from build123d import *

# Parameters (mm, degrees)
SKETCH_1_R          = 2
SKETCH_1_W          = 3
SKETCH_1_H          = 10
EXTRUDE_1_DEPTH     = 3
SKETCH_2_W          = 3
SKETCH_2_H          = 60
EXTRUDE_2_DEPTH     = 31
SKETCH_3_W          = 25
SKETCH_3_H          = 3
EXTRUDE_3_DEPTH     = 5
SKETCH_4_W          = 10
SKETCH_4_H          = 3
SKETCH_4_W_2        = 6
SKETCH_4_W_3        = 3
SKETCH_4_H_2        = 10
CUT_EXTRUDE_1_DEPTH = 3
SKETCH_5_R          = 1
CUT_EXTRUDE_2_DEPTH = 3
FILLET_1_R          = 1


with BuildPart() as part:
    # 草图1 → 凸台-拉伸1 (new body)
    with BuildSketch(Plane.XY):
        Polygon((-5, 25), (-5, 28), (1, 28), (1, 25), (5, 25), (10, 25), (20, 25), (25, 25), (30, 25), (30, -25), (25, -25), (20, -25), (10, -25), (5, -25), (1, -25), (1, -28), (-5, -28), (-5, -25), (-9, -25), (-9, -28), (-15, -28), (-15, -25), (-20, -25), (-20, 25), (-15, 25), (-15, 28), (-9, 28), (-9, 25), align=None)
        with Locations((-11, 15)):
            Circle(SKETCH_1_R, mode=Mode.SUBTRACT)
        with Locations((-11, -15)):
            Circle(SKETCH_1_R, mode=Mode.SUBTRACT)
        with Locations((19, -15)):
            Circle(SKETCH_1_R, mode=Mode.SUBTRACT)
        with Locations((19, 15)):
            Circle(SKETCH_1_R, mode=Mode.SUBTRACT)
        with Locations((26.5, 15)):
            Rectangle(SKETCH_1_W, SKETCH_1_H, mode=Mode.SUBTRACT)
        with Locations((26.5, 0)):
            Rectangle(SKETCH_1_W, SKETCH_1_H, mode=Mode.SUBTRACT)
        with Locations((26.5, -15)):
            Rectangle(SKETCH_1_W, SKETCH_1_H, mode=Mode.SUBTRACT)
        with Locations((1.5, 0)):
            Rectangle(SKETCH_1_W, SKETCH_1_H, mode=Mode.SUBTRACT)
        with Locations((1.5, -15)):
            Rectangle(SKETCH_1_W, SKETCH_1_H, mode=Mode.SUBTRACT)
        with Locations((1.5, 15)):
            Rectangle(SKETCH_1_W, SKETCH_1_H, mode=Mode.SUBTRACT)
    extrude(amount=EXTRUDE_1_DEPTH)

    # 草图2 → 凸台-拉伸2 (add)
    with BuildSketch(Plane.ZY.offset(20)):
        with Locations((1.5, 0)):
            Rectangle(SKETCH_2_W, SKETCH_2_H)
    extrude(amount=EXTRUDE_2_DEPTH)

    # 草图3 → 凸台-拉伸3 (add)
    with BuildSketch(Plane(origin=(0, 25, 0), x_dir=(1, 0, 0), z_dir=(0, 1, 0))):
        with Locations((17.5, -1.5)):
            Rectangle(SKETCH_3_W, SKETCH_3_H)
    extrude_3 = extrude(amount=EXTRUDE_3_DEPTH)

    # 镜向1: 凸台-拉伸3 across plane
    add(extrude_3.mirror(Plane.ZX))

    # 草图4 → 切除-拉伸1 (cut)
    with BuildSketch(Plane.XY.offset(3)):
        with Locations((-43, 26.5)):
            Rectangle(SKETCH_4_W, SKETCH_4_H)
        with Locations((-29, 26.5)):
            Rectangle(SKETCH_4_W, SKETCH_4_H)
        with Locations((12, 26.5)):
            Rectangle(SKETCH_4_W_2, SKETCH_4_H)
        with Locations((22, 26.5)):
            Rectangle(SKETCH_4_W_2, SKETCH_4_H)
        with Locations((22, -26.5)):
            Rectangle(SKETCH_4_W_2, SKETCH_4_H)
        with Locations((12, -26.5)):
            Rectangle(SKETCH_4_W_2, SKETCH_4_H)
        with Locations((-29, -26.5)):
            Rectangle(SKETCH_4_W, SKETCH_4_H)
        with Locations((-43, -26.5)):
            Rectangle(SKETCH_4_W, SKETCH_4_H)
        with Locations((-47.5, 0)):
            Rectangle(SKETCH_4_W_3, SKETCH_4_H_2)
        with Locations((-47.5, 15)):
            Rectangle(SKETCH_4_W_3, SKETCH_4_H_2)
        with Locations((-47.5, -15)):
            Rectangle(SKETCH_4_W_3, SKETCH_4_H_2)
    extrude(amount=-CUT_EXTRUDE_1_DEPTH, mode=Mode.SUBTRACT)

    # 草图5 → 切除-拉伸2 (cut)
    with BuildSketch(Plane(origin=(0, 0, 0), x_dir=(-1, 0, 0), z_dir=(0, 0, -1))):
        with Locations((23, 22.6)):
            Circle(SKETCH_5_R)
        with Locations((41, 22.6)):
            Circle(SKETCH_5_R)
        with Locations((41, -22.6)):
            Circle(SKETCH_5_R)
        with Locations((23, -22.6)):
            Circle(SKETCH_5_R)
        with BuildLine():
            Line((2, 7.351919832), (2, -7.055869369))
            Line((2, -7.055869369), (2, -10.9658561))
            ThreePointArc((2, -10.9658561), (8.5, 0), (2, 10.9658561))
            Line((2, 10.9658561), (2, 7.351919832))
        make_face()
        Polygon((23, -15), (23, 15), (28.973451327, 0), align=None)
        Polygon((27, -20), (32, -7.444444444), (37, -20), align=None)
        Polygon((41, -15), (35.026548673, 0), (41, 15), align=None)
        Polygon((27, 20), (37, 20), (32, 7.444444444), align=None)
    extrude(amount=-CUT_EXTRUDE_2_DEPTH, mode=Mode.SUBTRACT)

    # 圆角1
    fillet_1_edges = [part.edges().sort_by_distance(p)[0] for p in [
        (-2, 10.9658561, 1.5),
        (-2, -10.9658561, 1.5),
        (-23, 15, 1.5),
        (-28.973451327, 0, 1.5),
        (-23, -15, 1.5),
        (-37, 20, 1.5),
        (-32, 7.444444444, 1.5),
        (-27, 20, 1.5),
        (-41, 15, 1.5),
        (-41, -15, 1.5),
        (-35.026548673, 0, 1.5),
        (-37, -20, 1.5),
        (-27, -20, 1.5),
        (-32, -7.444444444, 1.5),
    ]]
    fillet(fillet_1_edges, radius=FILLET_1_R)


solid = part.part
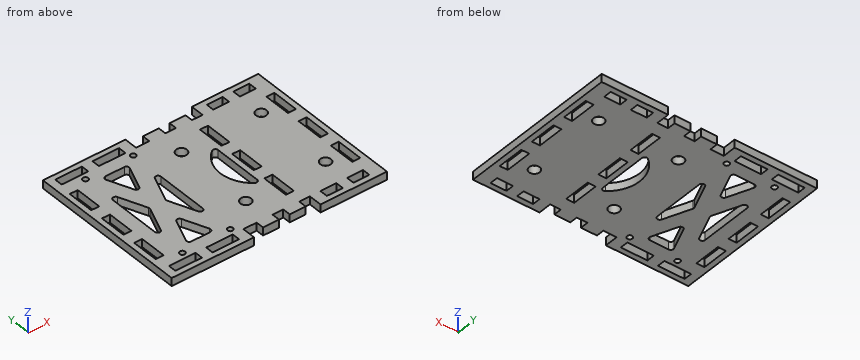
Part model, mm, in its own coordinate system. Round coordinates to 2 decimals unless told otherwise and drop trailing zeros. Write each loop counter-clockwise with the first axis right and the second up, starting at its lowest first coordinate (ties: lowest second). Pieces come first, ordered by that corner, then holes. Notation, with made-up numbers: (28, 81) - (47, 81) arc R13 ccw to (47, 104) - close; hole circle Ø9 at (11, 10). An arc over 180 degrees is marked (long way). Use CSV: the item, a comma, the result in double quotes.
Item 1: Slice it at A-A, the plane x = -11. Write the cut outline in (y, z).
Results list:
outline,"(-28, 0) - (-17, 0) - (-17, 3) - (-28, 3) - close; (-13, 0) - (13, 0) - (13, 3) - (-13, 3) - close; (17, 0) - (28, 0) - (28, 3) - (17, 3) - close"
Item 2: Wall check: L1, parallel to Y at x = 10, z = 0.9; L2, parallel to Y at x = -11, z = 2.05; L3, parallel to Y at x = 4, z = 2.2. Give the ranges that are in metal, low to high.
Results list:
L1,"y = -30 to -28, -25 to 25, 28 to 30"
L2,"y = -28 to -17, -13 to 13, 17 to 28"
L3,"y = -25 to 25"
Item 3: Slice it at C-C, the plane x = 12.5. Write the cut outline in (y, z), then the cut area to 3 significant figures.
Results list:
outline,"(-30, 0) - (-28, 0) - (-28, 3) - (-30, 3) - close; (-25, 0) - (25, 0) - (25, 3) - (-25, 3) - close; (28, 0) - (30, 0) - (30, 3) - (28, 3) - close"
area,"162 mm²"
Item 4: Flat gauge pin, fed straight in: P1, Ø0.9, axis at x = 1.5, z = 2, coming from the -Y side. Where does the tip first touch, or does it go through?
Results list:
P1,"stops at y = -25"
Item 5: Slice it at B-B, the plane y = 15. Write the cut outline in (x, z).
Results list:
outline,"(-51, 0) - (-49, 0) - (-49, 3) - (-51, 3) - close; (-46, 0) - (-35.01, 0) - (-35.01, 3) - (-46, 3) - close; (-28.99, 0) - (-13, 0) - (-13, 3) - (-28.99, 3) - close; (-9, 0) - (0, 0) - (0, 3) - (-9, 3) - close; (3, 0) - (17, 0) - (17, 3) - (3, 3) - close; (21, 0) - (25, 0) - (25, 3) - (21, 3) - close; (28, 0) - (30, 0) - (30, 3) - (28, 3) - close"
Item 6: Slice it at D-D, the plane z = 1.9. Count the separate pieces of the cut face and the enclosed holes in it, then the cut area to 3 significant figures.
Results list:
separate pieces,"1"
enclosed holes,"30"
area,"3,770 mm²"
